```python
from build123d import *

# Parameters (mm, degrees)
SKETCH_1_W          = 80
SKETCH_1_H          = 90
EXTRUDE_1_DEPTH     = 3
SKETCH_2_R          = 1.65
CUT_EXTRUDE_1_DEPTH = 3
CUT_EXTRUDE_2_REACH = 5
SKETCH_3_R          = 1.65
SKETCH_3_W          = 50
SKETCH_3_H          = 20
SKETCH_3_W_2        = 20
SKETCH_3_H_2        = 30
FILLET_1_R          = 5
CUT_EXTRUDE_3_REACH = 5
SKETCH_4_R          = 1.7


with BuildPart() as part:
    # 草图1 → 凸台-拉伸1 (new body)
    with BuildSketch(Plane.XY):
        with Locations((5.850106622, 2.961375961)):
            Rectangle(SKETCH_1_W, SKETCH_1_H)
    extrude(amount=EXTRUDE_1_DEPTH)

    # 草图2 → 切除-拉伸1 (cut)
    with BuildSketch(Plane(origin=(0, 0, 0), x_dir=(-1, 0, 0), z_dir=(0, 0, -1))):
        with Locations((31.149893378, -39.038624039)):
            Circle(SKETCH_2_R)
        with Locations((-42.850106622, -39.038624039)):
            Circle(SKETCH_2_R)
        with Locations((31.149893378, 44.961375961)):
            Circle(SKETCH_2_R)
        with Locations((-42.850106622, 44.961375961)):
            Circle(SKETCH_2_R)
    extrude(amount=-CUT_EXTRUDE_1_DEPTH, mode=Mode.SUBTRACT)

    # 草图3 → 切除-拉伸2 (cut, up to next)
    with BuildSketch(Plane(origin=(0, 0, 0), x_dir=(-1, 0, 0), z_dir=(0, 0, -1)), mode=Mode.PRIVATE) as cut_extrude_2_sk1:
        with Locations((-37.350106622, 24.461375961)):
            Circle(SKETCH_3_R)
    cut_extrude_2_tool1 = extrude(cut_extrude_2_sk1.sketch, amount=-CUT_EXTRUDE_2_REACH, mode=Mode.PRIVATE) & part.part
    add(cut_extrude_2_tool1.solids().sort_by_distance((37.350107, 24.461376, 0))[0], mode=Mode.SUBTRACT)
    # 草图3 → 切除-拉伸2 (cut, up to next)
    with BuildSketch(Plane(origin=(0, 0, 0), x_dir=(-1, 0, 0), z_dir=(0, 0, -1)), mode=Mode.PRIVATE) as cut_extrude_2_sk2:
        with Locations((25.649893378, 24.461375961)):
            Circle(SKETCH_3_R)
    cut_extrude_2_tool2 = extrude(cut_extrude_2_sk2.sketch, amount=-CUT_EXTRUDE_2_REACH, mode=Mode.PRIVATE) & part.part
    add(cut_extrude_2_tool2.solids().sort_by_distance((-25.649893, 24.461376, 0))[0], mode=Mode.SUBTRACT)
    # 草图3 → 切除-拉伸2 (cut, up to next)
    with BuildSketch(Plane(origin=(0, 0, 0), x_dir=(-1, 0, 0), z_dir=(0, 0, -1)), mode=Mode.PRIVATE) as cut_extrude_2_sk3:
        with Locations((25.649893378, -18.538624039)):
            Circle(SKETCH_3_R)
    cut_extrude_2_tool3 = extrude(cut_extrude_2_sk3.sketch, amount=-CUT_EXTRUDE_2_REACH, mode=Mode.PRIVATE) & part.part
    add(cut_extrude_2_tool3.solids().sort_by_distance((-25.649893, -18.538624, 0))[0], mode=Mode.SUBTRACT)
    # 草图3 → 切除-拉伸2 (cut, up to next)
    with BuildSketch(Plane(origin=(0, 0, 0), x_dir=(-1, 0, 0), z_dir=(0, 0, -1)), mode=Mode.PRIVATE) as cut_extrude_2_sk4:
        with Locations((-37.350106622, -18.538624039)):
            Circle(SKETCH_3_R)
    cut_extrude_2_tool4 = extrude(cut_extrude_2_sk4.sketch, amount=-CUT_EXTRUDE_2_REACH, mode=Mode.PRIVATE) & part.part
    add(cut_extrude_2_tool4.solids().sort_by_distance((37.350107, -18.538624, 0))[0], mode=Mode.SUBTRACT)
    # 草图3 → 切除-拉伸2 (cut, up to next)
    with BuildSketch(Plane(origin=(0, 0, 0), x_dir=(-1, 0, 0), z_dir=(0, 0, -1)), mode=Mode.PRIVATE) as cut_extrude_2_sk5:
        with Locations((-5.850106622, 37.961375961)):
            Rectangle(SKETCH_3_W, SKETCH_3_H)
    cut_extrude_2_tool5 = extrude(cut_extrude_2_sk5.sketch, amount=-CUT_EXTRUDE_2_REACH, mode=Mode.PRIVATE) & part.part
    add(cut_extrude_2_tool5.solids().sort_by_distance((5.850107, 37.961376, 0))[0], mode=Mode.SUBTRACT)
    # 草图3 → 切除-拉伸2 (cut, up to next)
    with BuildSketch(Plane(origin=(0, 0, 0), x_dir=(-1, 0, 0), z_dir=(0, 0, -1)), mode=Mode.PRIVATE) as cut_extrude_2_sk6:
        with Locations((-5.850106622, -32.038624039)):
            Rectangle(SKETCH_3_W, SKETCH_3_H)
    cut_extrude_2_tool6 = extrude(cut_extrude_2_sk6.sketch, amount=-CUT_EXTRUDE_2_REACH, mode=Mode.PRIVATE) & part.part
    add(cut_extrude_2_tool6.solids().sort_by_distance((5.850107, -32.038624, 0))[0], mode=Mode.SUBTRACT)
    # 草图3 → 切除-拉伸2 (cut, up to next)
    with BuildSketch(Plane(origin=(0, 0, 0), x_dir=(-1, 0, 0), z_dir=(0, 0, -1)), mode=Mode.PRIVATE) as cut_extrude_2_sk7:
        with Locations((24.149893378, 2.961375961)):
            Rectangle(SKETCH_3_W_2, SKETCH_3_H_2)
    cut_extrude_2_tool7 = extrude(cut_extrude_2_sk7.sketch, amount=-CUT_EXTRUDE_2_REACH, mode=Mode.PRIVATE) & part.part
    add(cut_extrude_2_tool7.solids().sort_by_distance((-24.149893, 2.961376, 0))[0], mode=Mode.SUBTRACT)
    # 草图3 → 切除-拉伸2 (cut, up to next)
    with BuildSketch(Plane(origin=(0, 0, 0), x_dir=(-1, 0, 0), z_dir=(0, 0, -1)), mode=Mode.PRIVATE) as cut_extrude_2_sk8:
        with Locations((-35.850106622, 2.961375961)):
            Rectangle(SKETCH_3_W_2, SKETCH_3_H_2)
    cut_extrude_2_tool8 = extrude(cut_extrude_2_sk8.sketch, amount=-CUT_EXTRUDE_2_REACH, mode=Mode.PRIVATE) & part.part
    add(cut_extrude_2_tool8.solids().sort_by_distance((35.850107, 2.961376, 0))[0], mode=Mode.SUBTRACT)

    # 圆角1
    fillet_1_edges = [part.edges().sort_by_distance(p)[0] for p in [
        (30.850106622, 47.961375961, 1.5),
        (-19.149893378, 47.961375961, 1.5),
        (-19.149893378, 27.961375961, 1.5),
        (30.850106622, 27.961375961, 1.5),
        (45.850106622, -12.038624039, 1.5),
        (45.850106622, 17.961375961, 1.5),
        (25.850106622, 17.961375961, 1.5),
        (25.850106622, -12.038624039, 1.5),
        (-14.149893378, 17.961375961, 1.5),
        (-34.149893378, 17.961375961, 1.5),
        (-34.149893378, -12.038624039, 1.5),
        (-14.149893378, -12.038624039, 1.5),
        (30.850106622, -22.038624039, 1.5),
        (-19.149893378, -22.038624039, 1.5),
        (-19.149893378, -42.038624039, 1.5),
        (30.850106622, -42.038624039, 1.5),
    ]]
    fillet(fillet_1_edges, radius=FILLET_1_R)

    # 草图4 → 切除-拉伸3 (cut, up to next)
    with BuildSketch(Plane(origin=(0, 0, 0), x_dir=(-1, 0, 0), z_dir=(0, 0, -1)), mode=Mode.PRIVATE) as cut_extrude_3_sk1:
        with Locations((3.649893378, 12.461375961)):
            Circle(SKETCH_4_R)
    cut_extrude_3_tool1 = extrude(cut_extrude_3_sk1.sketch, amount=-CUT_EXTRUDE_3_REACH, mode=Mode.PRIVATE) & part.part
    add(cut_extrude_3_tool1.solids().sort_by_distance((-3.649893, 12.461376, 0))[0], mode=Mode.SUBTRACT)
    # 草图4 → 切除-拉伸3 (cut, up to next)
    with BuildSketch(Plane(origin=(0, 0, 0), x_dir=(-1, 0, 0), z_dir=(0, 0, -1)), mode=Mode.PRIVATE) as cut_extrude_3_sk2:
        with Locations((3.649893378, -6.538624039)):
            Circle(SKETCH_4_R)
    cut_extrude_3_tool2 = extrude(cut_extrude_3_sk2.sketch, amount=-CUT_EXTRUDE_3_REACH, mode=Mode.PRIVATE) & part.part
    add(cut_extrude_3_tool2.solids().sort_by_distance((-3.649893, -6.538624, 0))[0], mode=Mode.SUBTRACT)
    # 草图4 → 切除-拉伸3 (cut, up to next)
    with BuildSketch(Plane(origin=(0, 0, 0), x_dir=(-1, 0, 0), z_dir=(0, 0, -1)), mode=Mode.PRIVATE) as cut_extrude_3_sk3:
        with Locations((-15.350106622, -6.538624039)):
            Circle(SKETCH_4_R)
    cut_extrude_3_tool3 = extrude(cut_extrude_3_sk3.sketch, amount=-CUT_EXTRUDE_3_REACH, mode=Mode.PRIVATE) & part.part
    add(cut_extrude_3_tool3.solids().sort_by_distance((15.350107, -6.538624, 0))[0], mode=Mode.SUBTRACT)
    # 草图4 → 切除-拉伸3 (cut, up to next)
    with BuildSketch(Plane(origin=(0, 0, 0), x_dir=(-1, 0, 0), z_dir=(0, 0, -1)), mode=Mode.PRIVATE) as cut_extrude_3_sk4:
        with Locations((-15.350106622, 12.461375961)):
            Circle(SKETCH_4_R)
    cut_extrude_3_tool4 = extrude(cut_extrude_3_sk4.sketch, amount=-CUT_EXTRUDE_3_REACH, mode=Mode.PRIVATE) & part.part
    add(cut_extrude_3_tool4.solids().sort_by_distance((15.350107, 12.461376, 0))[0], mode=Mode.SUBTRACT)


solid = part.part
```
For this review, take the finished solid that the model builds, in its own axes (mm). A direction names the side the tool comes from. Coordinates: 2 decimals unless noted, no trailing zeros. Write each loop counter-clockwise with the first axis right and the second up, starting at its lowest first coordinate (ties: lowest second). Pieces come first, ordered by that corner, then holes.
(1) The part is to be moulded in two halves that separate along Y. For faces 6 (the face through (-34.15, 35, 1)), 7 (the face through (29.42, -23.54, 1.52)), 8 (the face through (36, 17.961, 1)), say which applies: +Y half, -Y half, draft (parallel to the pull), parting line (faces both ways), or undercut.
(2) Add section C-C on x = 11. Give the boundary of the cut face in (y, z).
(3) Tool access review of faces 1 (the face through (30.85, -32, 1)), 2 (the face through (-34.15, -30, 1)), 3 (the face through (29.35, 29.39, 1.52)), 4 (the face through (25.85, 3, 1)), 5 (the face through (-32.65, 19.39, 1.52)): name each direction out of +Z, -Z, +X, -X, +Y, -Y from which nothing blocks a thin tool from reaching the whole face with its end or side.
(4) Add section D-D on y = 3. Give the boundary of the cut face in (x, z).
(5) Wall thickness on probe 1 along X at (y, z) = (12, 1); probe 2 along Y at (x, z) = (13, 1.5); probe 3 along X at (y, z) = (-5.5, 0.9): over which ranges is each line inside the solid? List them lowest first.
(6) Add section B-B on x = 29.5. Give the boundary of the cut face in (y, z), then the cut area to 3 significant figures.
(7) Add section A-A on y = -32. Give the boundary of the cut face in (x, z).
(8) For pin 1 Ø1 at (x, z) = (-23.5, 2.5) entering from -Y; pin 2 Ø1 at (x, z) = (-6, 1) entering from -Y; pin 3 Ø0.9 at (x, z) = (-22, 1) entering from +Y, all flat-tipped, find the tip position at first contact; note any pin that passes through.
Answer sheet:
1. face 6: draft
1. face 7: -Y half
1. face 8: undercut
2. outline: (-22.04, 0) - (27.96, 0) - (27.96, 3) - (-22.04, 3) - close
3. face 1: +Z, -Z, -Y
3. face 2: +Z, -Z, -X, +Y, -Y
3. face 3: +Z, -Z, +Y
3. face 4: +Z, -Z, +X
3. face 5: +Z, -Z, -X
4. outline: (-14.15, 0) - (25.85, 0) - (25.85, 3) - (-14.15, 3) - close
5. probe 1: x = -14.15 to -5.29, -2.01 to 13.71, 16.99 to 25.85
5. probe 2: y = -22.04 to 27.96
5. probe 3: x = -14.15 to -5, -2.3 to 14, 16.7 to 25.85
6. outline: (-23.62, 0) - (-11.85, 0) - (-11.85, 3) - (-23.62, 3) - close; (17.78, 0) - (29.54, 0) - (29.54, 3) - (17.78, 3) - close
6. area: 70.6 mm2
7. outline: (-34.15, 0) - (-19.15, 0) - (-19.15, 3) - (-34.15, 3) - close; (30.85, 0) - (45.85, 0) - (45.85, 3) - (30.85, 3) - close
8. pin 1: stops at y = -42.04
8. pin 2: stops at y = -22.04
8. pin 3: stops at y = 47.66
